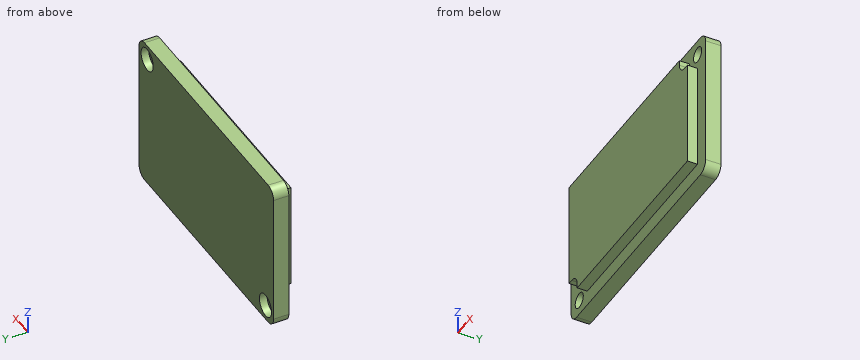
from build123d import *

# Parameters (mm, degrees)
CROQUIS2_W              = 50
CROQUIS2_H              = 30
SALIENTE_EXTRUIR2_DEPTH = 3
SALIENTE_EXTRUIR3_DEPTH = 2
REDONDEO1_R             = 2
CROQUIS6_R              = 1.5
CORTAR_EXTRUIR2_DEPTH   = 7
REDONDEO3_R             = 2
CROQUIS7_R              = 2.25
CORTAR_EXTRUIR3_DEPTH   = 1.5


with BuildPart() as part:
    # Croquis2 → Saliente-Extruir2 (new body)
    with BuildSketch(Plane(origin=(0, 0, 0), x_dir=(1, 0, 0), z_dir=(0, 1, 0))):
        Rectangle(CROQUIS2_W, CROQUIS2_H)
    extrude(amount=SALIENTE_EXTRUIR2_DEPTH)

    # Croquis3 → Saliente-Extruir3 (add)
    with BuildSketch(Plane.XZ):
        Polygon((-19, -12), (22, -12), (22, 9), (19, 9), (19, 12), (-22, 12), (-22, -9), (-19, -9), align=None)
    extrude(amount=SALIENTE_EXTRUIR3_DEPTH)

    # Redondeo1
    redondeo1_edges = [part.edges().sort_by_distance(p)[0] for p in [
        (25, 1.5, 15),
        (-25, 1.5, 15),
        (-25, 1.5, -15),
        (25, 1.5, -15),
    ]]
    fillet(redondeo1_edges, radius=REDONDEO1_R)

    # Croquis6 → Cortar-Extruir2 (cut)
    with BuildSketch(Plane.XZ):
        with Locations(Location((-22, -12, 0), (0, 0, 270))):
            Circle(CROQUIS6_R)
        with Locations(Location((22, 12, 0), (0, 0, 270))):
            Circle(CROQUIS6_R)
    extrude(amount=-CORTAR_EXTRUIR2_DEPTH, mode=Mode.SUBTRACT)

    # Redondeo3
    redondeo3_edges = [part.edges().sort_by_distance(p)[0] for p in [
        (-19, -1, -9),
        (19, -1, 9),
    ]]
    fillet(redondeo3_edges, radius=REDONDEO3_R)

    # Croquis7 → Cortar-Extruir3 (cut)
    with BuildSketch(Plane(origin=(0, 3, 0), x_dir=(1, 0, 0), z_dir=(0, 1, 0))):
        with Locations(Location((-22, 12, 0), (0, 0, 270))):
            Circle(CROQUIS7_R)
        with Locations(Location((22, -12, 0), (0, 0, 270))):
            Circle(CROQUIS7_R)
    extrude(amount=-CORTAR_EXTRUIR3_DEPTH, mode=Mode.SUBTRACT)


solid = part.part
For this review, take the finished solid that the model builds, in its own axes (mm). Round coordinates to 2 decimals unless told otherwise and drop trailing zeros. Write each loop counter-clockwise with the first axis right and the second up, starting at its lowest first coordinate (ties: lowest second). Pieces come first, ordered by that corner, then holes. Notation, with made-up numbers: (19.5, 9) -> (55.5, 9) arc R30 cw to (55.5, 40) -> close; hole circle Ø11 at (8, 26.25). An arc over 180 degrees is marked (long way). Use CSV: the item, a comma, the result in double quotes.
(1) To check wall thickness, follow L1, parallel to X at y = 2.1, z = 12; L2, parallel to X at y = 2.6, z = -12; L3, parallel to Z at x = -3.5, y = -0.15. State the ranges of each line that lie inside material, in increasing order. Write a range as [from, to].
Computed values:
L1,"[-25, 19.75], [24.25, 25]"
L2,"[-25, -24.25], [-19.75, 25]"
L3,"[-12, 12]"
(2) Consider section C-C, the plane y = -1.1. Give the boundary of the cut face in (x, z), plus the area to 3 significant figures.
Computed values:
outline,"(-22, -9) -> (-21, -9) arc R2 cw to (-19, -11) -> (-19, -12) -> (22, -12) -> (22, 9) -> (21, 9) arc R2 cw to (19, 11) -> (19, 12) -> (-22, 12) -> close"
area,"1,040 mm²"
(3) Consider section A-A, the plane y = 2.1. Give the boundary of the cut face in (x, z).
Computed values:
outline,"(-25, -13) arc R2 ccw to (-23, -15) -> (23, -15) arc R2 ccw to (25, -13) -> (25, 13) arc R2 ccw to (23, 15) -> (-23, 15) arc R2 ccw to (-25, 13) -> close; hole circle Ø4.5 at (-22, -12); hole circle Ø4.5 at (22, 12)"
(4) Consider section D-D, the plane x = -8.5. Give the boundary of the cut face in (y, z).
Computed values:
outline,"(-2, -12) -> (0, -12) -> (0, -15) -> (3, -15) -> (3, 15) -> (0, 15) -> (0, 12) -> (-2, 12) -> close"
(5) Consider section B-B, the plane z = 8.5. Give the boundary of the cut face in (x, y), plus the area to 3 significant figures.
Computed values:
outline,"(-25, 0) -> (-22, 0) -> (-22, -2) -> (22, -2) -> (22, 0) -> (25, 0) -> (25, 3) -> (-25, 3) -> close"
area,"238 mm²"
(6) Clearance check with flat-ended pins moving along their axes: P1, Ø0.5, axis at y = -1, z = 11.5, coming from the +X side; P2, Ø4, axis at x = 22, z = 12, coming from the +Y side; P3, Ø0.6, axis at y = -1.5, z = -1, coming from the +X side. State where each tip first meets the part, or that it passes through.
Computed values:
P1,"x = 19"
P2,"y = 1.5"
P3,"x = 22"
